Geometry check sheet. Reference: drawing and pictorial views, mm from the part's lowest x, y, z. A direction names the side the tool comes from. Give positions to 0.01 mm unless a question says otherwise; leave off trailing zeros. Order: outer loops, then holes, each group sorted by start corner. A loop starts at its lowest first (then second) coordinate and runs counter-clockwise, first axis right, second up. Notation, with made-up numbers: (-30.75, 77) -> (4.25, 77) arc R9 cw to (4.25, 88) -> close; hole circle Ø5 at (28.25, 43.25). An arc over 180 degrees is marked (long way). Write each question's results on one line, items separated by ' | '.
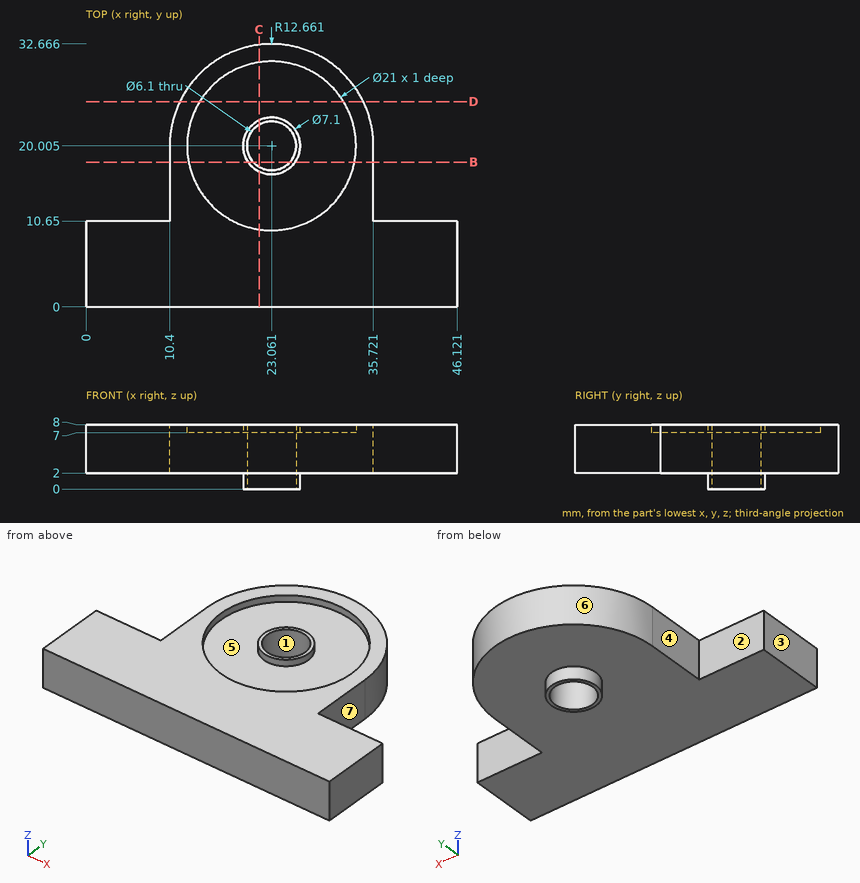
1. Mould release check, pull along X, two halves, no side actions. Record for the marked faces 1, 2 and 3: +X half, -X half, draft (parallel to the pull), parting line (faces both ways), or undercut.
Verdict:
face 1: undercut | face 2: draft | face 3: -X half
2. Access from +Z, -Z, +X, -X, +Y, -Y to the whole of each face (thin tool, end or side, straight path). Record for the marked faces 4, 5, 6 and 7.
Verdict:
face 4: +Z, -Z, -X, +Y | face 5: +Z | face 6: +Z, -Z, +Y | face 7: +Z, -Z, +X, +Y
3. Section check C-C on x = 21.5. Record the cut outline in (y, z) (1 decimal).
Verdict:
outline: (0, 2) -> (16.8, 2) -> (16.8, 0) -> (17.4, 0) -> (17.4, 8) -> (16.8, 8) -> (16.8, 7) -> (9.6, 7) -> (9.6, 8) -> (0, 8) -> close; (22.6, 0) -> (23.2, 0) -> (23.2, 2) -> (32.6, 2) -> (32.6, 8) -> (30.4, 8) -> (30.4, 7) -> (23.2, 7) -> (23.2, 8) -> (22.6, 8) -> close
4. Section check B-B on y = 18. Record the cut outline in (x, z), then the cut area to 3 significant figures.
Verdict:
outline: (10.4, 2) -> (20.13, 2) -> (20.13, 0) -> (20.76, 0) -> (20.76, 8) -> (20.13, 8) -> (20.13, 7) -> (12.75, 7) -> (12.75, 8) -> (10.4, 8) -> close; (25.36, 0) -> (25.99, 0) -> (25.99, 2) -> (35.72, 2) -> (35.72, 8) -> (33.37, 8) -> (33.37, 7) -> (25.99, 7) -> (25.99, 8) -> (25.36, 8) -> close | area: 112 mm^2
5. Section check D-D on y = 25.5. Record the cut outline in (x, z) (1 decimal).
Verdict:
outline: (11.7, 2) -> (34.5, 2) -> (34.5, 8) -> (32, 8) -> (32, 7) -> (14.1, 7) -> (14.1, 8) -> (11.7, 8) -> close
6. Gauge pin test, flat ends, axial feed: pin 1 Ø16.5 at (x, y) = (26, 12.5) entering from -Z; pin 2 Ø2 at (y, z) = (18, 2) entering from -X; pin 3 Ø1.8 at (x, z) = (6, 4) entering from +Y; pin 4 Ø1.8 at (y, z) = (15.5, 4.5) entering from +X. Record the tip position at first contact, or that the pin passes through.
Verdict:
pin 1: stops at z = 0 | pin 2: stops at x = 10.4 | pin 3: stops at y = 10.65 | pin 4: stops at x = 35.72
7. Material ranges on probe 1 along Z at (x, y) = (40, 8.5); probe 2 along Y at (x, z) = (44, 5.75); probe 3 along Z at (x, y) = (21.5, 27), recorded low to high. Write a range as from..to.
Verdict:
probe 1: z = 2..8 | probe 2: y = 0..10.65 | probe 3: z = 2..7
